from build123d import *

# Parameters (mm, degrees)
F0_R      = 9.5
F1_DEPTH  = 6
F2_R      = 7.8
F3_DEPTH  = 1.2
F4_R      = 7.8
F5_DEPTH  = 1.2
F6_R      = 4
F7_DEPTH  = 6
F8_R      = 2
F9_R      = 3.875
F10_DEPTH = 8.401
F11_SIZE  = 1


# Not quite as in the source:
# - the program builds the solid bodies; features that only make, move or delete a surface that nothing else refers to are left out


with BuildPart() as f1:
    # F0 (on Top) → F1 (new body)
    with BuildSketch(Plane.XY):
        Circle(F0_R)
    extrude(amount=F1_DEPTH)

    # F2 (on face) → F3 (join)
    with BuildSketch(Plane.XY.offset(6)):
        Circle(F2_R)
    extrude(amount=F3_DEPTH)

    # F4 (on face) → F5 (join)
    with BuildSketch(Plane(origin=(0, 0, 0), x_dir=(1, 0, 0), z_dir=(0, 0, -1))):
        Circle(F4_R)
    extrude(amount=F5_DEPTH)

    # F6 (on face) → F7 (cut, through all)
    with BuildSketch(Plane(origin=(0, 0, 0), x_dir=(1, 0, 0), z_dir=(0, 0, -1))):
        with Locations((0, 12.5)):
            Circle(F6_R)
        with Locations((-8.8388347648, 8.8388347648)):
            Circle(F6_R)
        with Locations((-12.5, 0)):
            Circle(F6_R)
        with Locations((-8.8388347648, -8.8388347648)):
            Circle(F6_R)
        with Locations((0, -12.5)):
            Circle(F6_R)
        with Locations((8.8388347648, -8.8388347648)):
            Circle(F6_R)
        with Locations((12.5, 0)):
            Circle(F6_R)
        with Locations((8.8388347648, 8.8388347648)):
            Circle(F6_R)
    extrude(amount=-F7_DEPTH, mode=Mode.SUBTRACT)

    # F8
    f8_edges = [f1.edges().sort_by_distance(p)[0] for p in [
        (-9.22, -2.289454, 3),
        (-9.22, 2.289454, 3),
        (-4.900636, -8.138413, 3),
        (-8.138413, -4.900636, 3),
        (-8.138413, 4.900636, 3),
        (-4.900636, 8.138413, 3),
        (-2.289454, 9.22, 3),
        (2.289454, 9.22, 3),
        (8.138413, 4.900636, 3),
        (4.900636, 8.138413, 3),
        (9.22, 2.289454, 3),
        (9.22, -2.289454, 3),
        (8.138413, -4.900636, 3),
        (4.900636, -8.138413, 3),
        (2.289454, -9.22, 3),
        (-2.289454, -9.22, 3),
    ]]
    fillet(f8_edges, radius=F8_R)

    # F9 (on face) → F10 (cut, through all)
    with BuildSketch(Plane.XY.offset(7.2)):
        Circle(F9_R)
    extrude(amount=-F10_DEPTH, mode=Mode.SUBTRACT)

    # F11
    f11_edges = [f1.edges().sort_by_distance(p)[0] for p in [
        (-3.875, 0, 7.2),
        (-3.875, 0, -1.2),
    ]]
    chamfer(f11_edges, length=F11_SIZE)


solid = f1.part
For this review, take the finished solid that the model builds, in its own axes (mm). A direction names the side the tool comes from. Round coordinates to 2 decimals unless told otherwise and drop trailing zeros. Write each loop counter-clockwise with the first axis right and the second up, starting at its lowest first coordinate (ties: lowest second). Pieces come first, ordered by that corner, then holes. Notation, with made-up numbers: (64.25, 49.5) - (123.25, 49.5) arc R18 ccw to (123.25, 57.5) - close; hole circle Ø7 at (-16, 83.25). An arc over 180 degrees is marked (long way). Write item = value, one per line. Start each with the question number.
1. For faces 4 (the face through (-3.63, 8.78, 2.96)), 5 (the face through (-4, 7, 6)), 6 (the face through (-4, 7, 0)), list the 3-axis set-ups (+Z, -Z, +X, -X, +Y, -Y) from which the entire face can be reached by the end or side of a thin tool; tool diameter is ignored.
2. Consider section A-A on y = 0. State the section outline as (x, z) points (3 decimals), plus the area to 3 significant figures.
3. For pin 1 Ø1.5 at (x, y) = (6, -6.5) entering from +Z; pin 2 Ø9 at (x, y) = (0, 0) entering from -Z (3 decimals); pin 3 Ø1.5 at (x, z) = (5, 5) entering from +Y, all flat-tipped, find the tip position at first contact; note any pin that passes through.
4. Draft analysis for pull direction X (two halves, no side actions). For faces 1 (the face through (3.63, -8.78, 2.96)), 2 (the face through (0, -8.5, 3)), 3 (the face through (-0.1, 5.1, -1.2)), state which applies: released by +X, released by -X, zero draft, split by the parting line, or undercut.
5. Consider section C-C on x = -5.5. State the section outline as (y, z) points.
6. Wall thickness on L1, parallel to X at y = -1.25, z = 3; L2, parallel to Y at x = -1.75, z = 2; L3, parallel to Z at x = 8, y = -0.25: over which ranges is each line inside the solid? List them lowest first.
Evaluation:
q1.face_4 = +Z, -Z, -X, +Y
q1.face_5 = +Z
q1.face_6 = -Z
q2.outline = (-8.5, 0) - (-7.8, 0) - (-7.8, -1.2) - (-4.875, -1.2) - (-3.875, -0.2) - (-3.875, 6.2) - (-4.875, 7.2) - (-7.8, 7.2) - (-7.8, 6) - (-8.5, 6) - close; (3.875, -0.2) - (4.875, -1.2) - (7.8, -1.2) - (7.8, 0) - (8.5, 0) - (8.5, 6) - (7.8, 6) - (7.8, 7.2) - (4.875, 7.2) - (3.875, 6.2) - close
q2.area = 72.3 mm2
q3.pin_1 = 6
q3.pin_2 = -0.825
q3.pin_3 = 8.49
q4.face_1 = released by +X
q4.face_2 = undercut
q4.face_3 = zero draft
q5.outline = (-6.64, 0) - (-5.53, 0) - (-5.53, -1.2) - (5.53, -1.2) - (5.53, 0) - (6.64, 0) - (6.64, 6) - (5.53, 6) - (5.53, 7.2) - (-5.53, 7.2) - (-5.53, 6) - (-6.64, 6) - close
q6.L1 = -8.7 to -3.67, 3.67 to 8.7
q6.L2 = -8.9 to -3.46, 3.46 to 8.9
q6.L3 = 0 to 6
